Work out the finished part from the listing and answer in its coordinate system (mm). Coordinates: 2 decimals unless noted, no trailing zeros. Loops run counter-clockwise (first coordinate to the right, second up) from the corner with the lowest first, then second, coordinate; pieces in that order, holes last. Notation, with made-up numbers: (10, -26) -> (32, -26) arc R31 ccw to (32, 2) -> close; hole circle Ø3 at (74.5, 10.25). An arc over 180 degrees is marked (long way). Use a Markdown table: item, result.
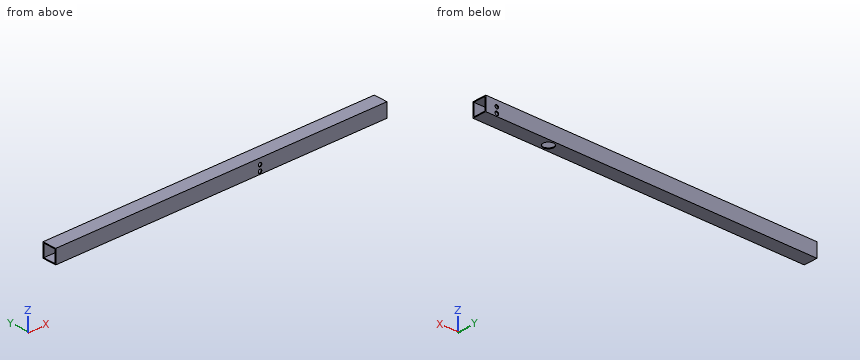
from build123d import *

# Parameters (mm, degrees)
SKETCH1_W           = 50
SKETCH1_H           = 50
SKETCH1_W_2         = 44
SKETCH1_H_2         = 44
BOSS_EXTRUDE1_DEPTH = 1200
CUT_EXTRUDE1_REACH  = 1203.301
SKETCH2_R           = 19
CUT_EXTRUDE2_REACH  = 1203.301
SKETCH3_R           = 6.5
CIRPATTERN1_COUNT   = 2


with BuildPart() as part:
    # Sketch1 → Boss-Extrude1 (new body)
    with BuildSketch(Plane(origin=(0, 0, 0), x_dir=(0, 0, -1), z_dir=(1, 0, 0))):
        Rectangle(SKETCH1_W, SKETCH1_H)
        Rectangle(SKETCH1_W_2, SKETCH1_H_2, mode=Mode.SUBTRACT)
    extrude(amount=BOSS_EXTRUDE1_DEPTH)

    # Sketch2 → Cut-Extrude1 (cut, up to next)
    with BuildSketch(Plane(origin=(0, 0, -25), x_dir=(-1, 0, 0), z_dir=(0, 0, -1)), mode=Mode.PRIVATE) as cut_extrude1_sk1:
        with Locations(Location((-950, 0, 0), (0, 0, 90))):
            Circle(SKETCH2_R)
    cut_extrude1_tool1 = extrude(cut_extrude1_sk1.sketch, amount=-CUT_EXTRUDE1_REACH, mode=Mode.PRIVATE) & part.part
    add(cut_extrude1_tool1.solids().sort_by_distance((950, 0, -25))[0], mode=Mode.SUBTRACT)

    # Sketch3 → Cut-Extrude2 (cut, up to next)
    with BuildSketch(Plane(origin=(0, 25, 0), x_dir=(1, 0, 0), z_dir=(0, 1, 0)), mode=Mode.PRIVATE) as cut_extrude2_sk1:
        with Locations(Location((1160, -4.5, 0), (0, 0, 270))):
            Circle(SKETCH3_R)
    cut_extrude2_tool1 = extrude(cut_extrude2_sk1.sketch, amount=-CUT_EXTRUDE2_REACH, mode=Mode.PRIVATE) & part.part
    # Sketch3 → Cut-Extrude2 (cut, up to next)
    with BuildSketch(Plane(origin=(0, 25, 0), x_dir=(1, 0, 0), z_dir=(0, 1, 0)), mode=Mode.PRIVATE) as cut_extrude2_sk2:
        with Locations(Location((1160, 15.5, 0), (0, 0, 270))):
            Circle(SKETCH3_R)
    cut_extrude2_tool2 = extrude(cut_extrude2_sk2.sketch, amount=-CUT_EXTRUDE2_REACH, mode=Mode.PRIVATE) & part.part
    cut_extrude2_1 = cut_extrude2_tool1.solids().sort_by_distance((1160, 25, 4.5))[0]
    add(cut_extrude2_1, mode=Mode.SUBTRACT)
    cut_extrude2_2 = cut_extrude2_tool2.solids().sort_by_distance((1160, 25, -15.5))[0]
    add(cut_extrude2_2, mode=Mode.SUBTRACT)
    cut_extrude2 = cut_extrude2_1 + cut_extrude2_2  # Cut-Extrude2 as one shape, for the pattern or mirror that repeats it

    # CirPattern1: Cut-Extrude2 ×2 about axis
    cirpattern1_axis = Axis((950, 0, 25.001), (0, 0, -1))
    for i in range(1, CIRPATTERN1_COUNT):
        add(cut_extrude2.rotate(cirpattern1_axis, i * 360 / CIRPATTERN1_COUNT), mode=Mode.SUBTRACT)


solid = part.part
Q1. Section A-A on y = 0 is taken. Determine the outline of the cut face in (x, z), and give its area (3 significant figures).
Solved:
| item | result |
|---|---|
| outline | (0, -25) -> (931, -25) -> (931, -22) -> (0, -22) -> close; (0, 22) -> (1200, 22) -> (1200, 25) -> (0, 25) -> close; (969, -25) -> (1200, -25) -> (1200, -22) -> (969, -22) -> close |
| area | 7,090 mm² |
Q2. Section C-C on x = 950 is taken. Determine the outline of the cut face in (y, z), and give its area (3 significant figures).
Solved:
| item | result |
|---|---|
| outline | (-25, -25) -> (-19, -25) -> (-19, -22) -> (-22, -22) -> (-22, 22) -> (22, 22) -> (22, -22) -> (19, -22) -> (19, -25) -> (25, -25) -> (25, 25) -> (-25, 25) -> close |
| area | 450 mm² |
Q3. Given pin 1 Ø10 at (y, z) = (-6, -15) entering from -X, flat-ended and moving along its own axis, determine where the tip first touches the part or whether it passes through.
Solved:
| item | result |
|---|---|
| pin 1 | through |
Q4. Section B-B on x = 654 is taken. Determine the outline of the cut face in (y, z), and give its area (3 significant figures).
Solved:
| item | result |
|---|---|
| outline | (-25, -25) -> (25, -25) -> (25, 25) -> (-25, 25) -> close; hole (-22, -22) -> (22, -22) -> (22, 22) -> (-22, 22) -> close |
| area | 564 mm² |
Q5. Consider line 1 (Z direction, x = 740, y = -23); line 2 (Y direction, x = 271.5, z = 15.5). Determine where each line is inside the solid, lowest interval first. Write a range as [from, to].
Solved:
| item | result |
|---|---|
| line 1 | [-25, -22], [-9, -2], [11, 25] |
| line 2 | [-25, -22], [22, 25] |
